from build123d import *

# Parameters (mm, degrees)
BOSS_EXTRUDE1_DEPTH = 80
SKETCH2_W           = 20
SKETCH2_H           = 10
BOSS_EXTRUDE2_DEPTH = 400
SKETCH3_W           = 20
SKETCH3_H           = 20
BOSS_EXTRUDE3_DEPTH = 400
BOSS_EXTRUDE4_DEPTH = 20
BOSS_EXTRUDE5_DEPTH = 20
SKETCH8_R           = 2.5
CUT_EXTRUDE1_DEPTH  = 20
CUT_EXTRUDE3_DEPTH  = 20


with BuildPart() as part:
    # Sketch1 → Boss-Extrude1 (new body)
    with BuildSketch(Plane(origin=(0, 0, 0), x_dir=(1, 0, 0), z_dir=(0, 1, 0))):
        with BuildLine():
            Line((-110, 0), (-100, 0))
            ThreePointArc((-100, 0), (0, 100), (100, 0))
            Line((100, 0), (110, 0))
            ThreePointArc((110, 0), (0, 110), (-110, 0))
        make_face()
    extrude(amount=BOSS_EXTRUDE1_DEPTH)

    # Sketch2 → Boss-Extrude2 (add)
    with BuildSketch(Plane(origin=(100, 80, 0), x_dir=(0, 0, 1), z_dir=(-1, 0, 0))):
        with Locations((-10, -35)):
            Rectangle(SKETCH2_W, SKETCH2_H)
        with Locations((-10, -45)):
            Rectangle(SKETCH2_W, SKETCH2_H)
    extrude(amount=-BOSS_EXTRUDE2_DEPTH)

    # Sketch3 → Boss-Extrude3 (add)
    with BuildSketch(Plane(origin=(-100, 80, 0), x_dir=(0, 0, -1), z_dir=(1, 0, 0))):
        with Locations((10, -40)):
            Rectangle(SKETCH3_W, SKETCH3_H)
    extrude(amount=-BOSS_EXTRUDE3_DEPTH)

    # Sketch5 → Boss-Extrude4 (add)
    with BuildSketch(Plane(origin=(0, 50, 0), x_dir=(1, 0, 0), z_dir=(0, 1, 0))):
        with BuildLine():
            Line((500, 0), (510, 0))
            ThreePointArc((510, 0), (504.329046943, 75.843341231), (487.442304278, 150))
            Line((487.442304278, 150), (476.969600708, 150))
            ThreePointArc((476.969600708, 150), (494.208862908, 75.878849641), (500, 0))
        make_face()
    extrude(amount=-BOSS_EXTRUDE4_DEPTH)

    # Sketch7 → Boss-Extrude5 (add)
    with BuildSketch(Plane(origin=(0, 50, 0), x_dir=(1, 0, 0), z_dir=(0, 1, 0))):
        with BuildLine():
            ThreePointArc((-510, 0), (-504.329046943, 75.843341231), (-487.442304278, 150))
            Line((-487.442304278, 150), (-476.969600708, 150))
            ThreePointArc((-476.969600708, 150), (-494.208862908, 75.878849641), (-500, 0))
            Line((-500, 0), (-510, 0))
        make_face()
    extrude(amount=-BOSS_EXTRUDE5_DEPTH)

    # Sketch8 → Cut-Extrude1 (cut)
    with BuildSketch(Plane(origin=(0, 0, -20), x_dir=(-1, 0, 0), z_dir=(0, 0, -1))):
        with Locations((-408.166538264, 40)):
            Circle(SKETCH8_R)
        with Locations((-258.166538264, 40)):
            Circle(SKETCH8_R)
        with Locations((258.166538264, 40)):
            Circle(SKETCH8_R)
        with Locations((408.166538264, 40)):
            Circle(SKETCH8_R)
        with Locations((-458.166538264, 40)):
            Circle(SKETCH8_R)
        with Locations((-208.166538264, 40)):
            Circle(SKETCH8_R)
        with Locations((208.166538264, 40)):
            Circle(SKETCH8_R)
        with Locations((458.166538264, 40)):
            Circle(SKETCH8_R)
    extrude(amount=-CUT_EXTRUDE1_DEPTH, mode=Mode.SUBTRACT)

    # Sketch9 → Cut-Extrude3 (cut)
    with BuildSketch(Plane(origin=(0, 80, -110), x_dir=(-1, 0, 0), z_dir=(0, 0, -1))):
        with BuildLine():
            ThreePointArc((0, -35), (-5, -40), (0, -45))
            Line((0, -45), (0, -35))
        make_face()
        with BuildLine():
            Line((0, -35), (0, -45))
            ThreePointArc((0, -45), (3.535533906, -43.535533906), (5, -40))
            ThreePointArc((5, -40), (3.535533906, -36.464466094), (0, -35))
        make_face()
    extrude(amount=-CUT_EXTRUDE3_DEPTH, mode=Mode.SUBTRACT)


solid = part.part
For this review, take the finished solid that the model builds, in its own axes (mm). A direction names the side the tool comes from. Give positions to 0.01 mm unless a question says otherwise; leave off trailing zeros. Loops run counter-clockwise (first coordinate to the right, second up) from the corner with the lowest first, then second, coordinate; pieces in that order, holes last. Notation, with made-up numbers: M -24,53 L -8,53 A15 ccw -8,57 Z; hole C 4.25,31 d6. An arc over 180 degrees is marked long. Answer as a JSON object with one key per item and string values. Group by question number.
Q1. Add section D-D on y = 64. Give the boundary of the cut face in (x, z), and give its area (3 significant figures).
Q2. Tool access review of faces 4 (the cylindrical face through (-492.432, 40.14, -86.662)), 5 (the flat face through (-337.9, 50, -19.8)), 6 (the flat face through (337.9, 50, -19.8)): name each direction out of +Z, -Z, +X, -X, +Y, -Y from which nothing blocks a thin tool from reaching the whole face with its end or side.
Q3. Insertion check: P1, Ø6, axis at y = 48, z = -134.5, coming from the -X side; P2, Ø3, axis at x = 16.5, y = 45.5, coming from the +Z side; P3, Ø8, axis at x = 208.17, y = 40, coming from the -Z side. Each pin has a flat end and moves straight along its axis. Give the tip position at first contact, or say it passes through.
Q4. Add section C-C on x = -151.5. Give the boundary of the cut face in (y, z), and give its area (3 significant figures).
Q5. Mouldability with a two-part tool opening along X and no side actions: class faces 1 (the flat face through (-301, 40, -20)), 2 (the flat face through (-9, 80, -100)), 3 (the cylindrical face through (-504.486, 40.14, -74.789)) as +X half, -X half, draft (parallel to the pull), parting line (faces both ways), or undercut.
Q6. Add section A-A on z = -139.5. Give the boundary of the cut face in (x, y), and give its area (3 significant figures).
Q7. For probe 1 along Y at (x, z) = (258.5, -11); probe 2 along X at (y, z) = (69.5, -60); probe 3 along Z at (x, y) = (433, 35.5), list the stretches that pass through material, from the lowest coordinate up. Write a range as [from, to].
Q8. Add section B-B on z = -36.5. Give the boundary of the cut face in (x, y).
Checked values:
{
 "1": {"outline": "M -110,0 A110 ccw 110,0 L 100,0 A100 cw -100,0 Z", "area": "3,300 mm²"},
 "2": {"face 4": "+Y, -Y", "face 5": "+Z, -Z, -X, +Y", "face 6": "+Z, -Z, +X, +Y"},
 "3": {"P1": "x = -492.76", "P2": "z = -98.37", "P3": "z = -20"},
 "4": {"outline": "M 30,-20 L 50,-20 L 50,0 L 30,0 Z", "area": "400 mm²"},
 "5": {"face 1": "undercut", "face 2": "draft", "face 3": "-X half"},
 "6": {"outline": "M -490.55,30 L -480.15,30 L -480.15,50 L -490.55,50 Z; M 480.15,30 L 490.55,30 L 490.55,50 L 480.15,50 Z", "area": "416 mm²"},
 "7": {"probe 1": "[30, 37.52], [42.48, 50]", "probe 2": "[-92.2, -80], [80, 92.2]", "probe 3": "[-20, 0]"},
 "8": {"outline": "M -508.69,30 L -498.67,30 L -498.67,50 L -508.69,50 Z; M -103.77,0 L -93.1,0 L -93.1,80 L -103.77,80 Z; M 93.1,0 L 103.77,0 L 103.77,80 L 93.1,80 Z; M 498.67,30 L 508.69,30 L 508.69,50 L 498.67,50 Z"}
}
